Verification items for this drawing (mm, ordinates from the low corner). Coordinates: 2 decimals unless noted, no trailing zeros. Write each loop counter-clockwise with the first axis right and the second up, starting at its lowest first coordinate (ties: lowest second). Pieces come first, ordered by that corner, then holes. Notation, with made-up numbers: (-10.5, 46.25) -> (44.5, 46.25) arc R30 cw to (44.5, 83.25) -> close; hole circle Ø2 at (-35, -31.75). An arc over 180 degrees is marked (long way). Answer as CSV lines item,"result".
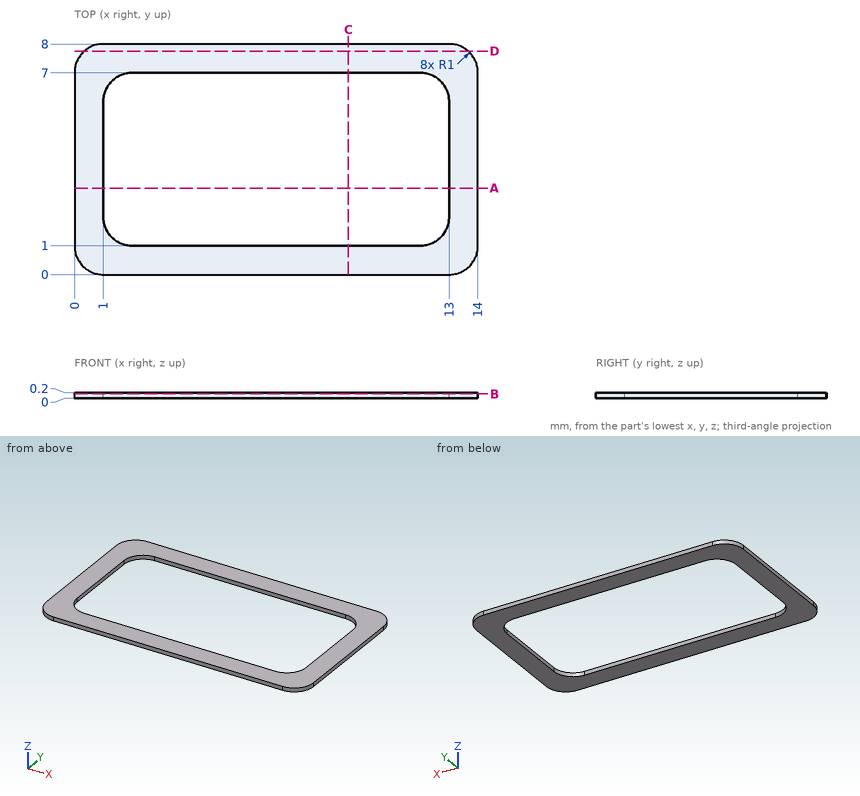
Item 1: Cross-section at A-A, the plane y = 3. Record the cut outline in (x, z).
Responses:
outline,"(0, 0) -> (1, 0) -> (1, 0.2) -> (0, 0.2) -> close; (13, 0) -> (14, 0) -> (14, 0.2) -> (13, 0.2) -> close"
Item 2: Cross-section at B-B, the plane z = 0.15. Record the cut outline in (x, y), plus the area to 3 significant figures.
Responses:
outline,"(0, 1) arc R1 ccw to (1, 0) -> (13, 0) arc R1 ccw to (14, 1) -> (14, 7) arc R1 ccw to (13, 8) -> (1, 8) arc R1 ccw to (0, 7) -> close; hole (1, 2) arc R1 ccw to (2, 1) -> (12, 1) arc R1 ccw to (13, 2) -> (13, 6) arc R1 ccw to (12, 7) -> (2, 7) arc R1 ccw to (1, 6) -> close"
area,"40.0 mm2"
Item 3: Thickness scan on probe 1 along X at (y, z) = (2.75, 0.1); probe 2 along Y at (x, z) = (9.5, 0.15); probe 3 along Y at (x, z) = (1.5, 0.1). Record the ranges inside material, lowest first.
Responses:
probe 1,"x = 0 to 1, 13 to 14"
probe 2,"y = 0 to 1, 7 to 8"
probe 3,"y = 0 to 1.13, 6.87 to 8"
Item 4: Depth check by flat-ended pin: pin 1 Ø3 at (x, y) = (10.5, 7) entering from -Z. Enter the tip coordinate at first touch or a pass-through.
Responses:
pin 1,"stops at z = 0"
Item 5: Cross-section at C-C, the plane x = 9.5. Record the cut outline in (y, z), plus the area to 3 significant figures.
Responses:
outline,"(0, 0) -> (1, 0) -> (1, 0.2) -> (0, 0.2) -> close; (7, 0) -> (8, 0) -> (8, 0.2) -> (7, 0.2) -> close"
area,"0.400 mm2"
Item 6: Cross-section at D-D, the plane y = 7.75. Record the cut outline in (x, z), plus the area to 3 significant figures.
Responses:
outline,"(0.34, 0) -> (13.66, 0) -> (13.66, 0.2) -> (0.34, 0.2) -> close"
area,"2.66 mm2"
